Can you work these out from the drawing? Everything is in mm from the part's minimum corner. Round coordinates to 2 decimals unless told otherwise and drop trailing zeros. Loops run counter-clockwise (first coordinate to the right, second up) from the corner with the lowest first, then second, coordinate; pieces in that order, holes last. Notation, with made-up numbers: (82.5, 39) -> (134.5, 39) arc R34 cw to (134.5, 72) -> close; hole circle Ø10 at (40, -33.75). An arc over 180 degrees is marked (long way). One line per item, written item: value.
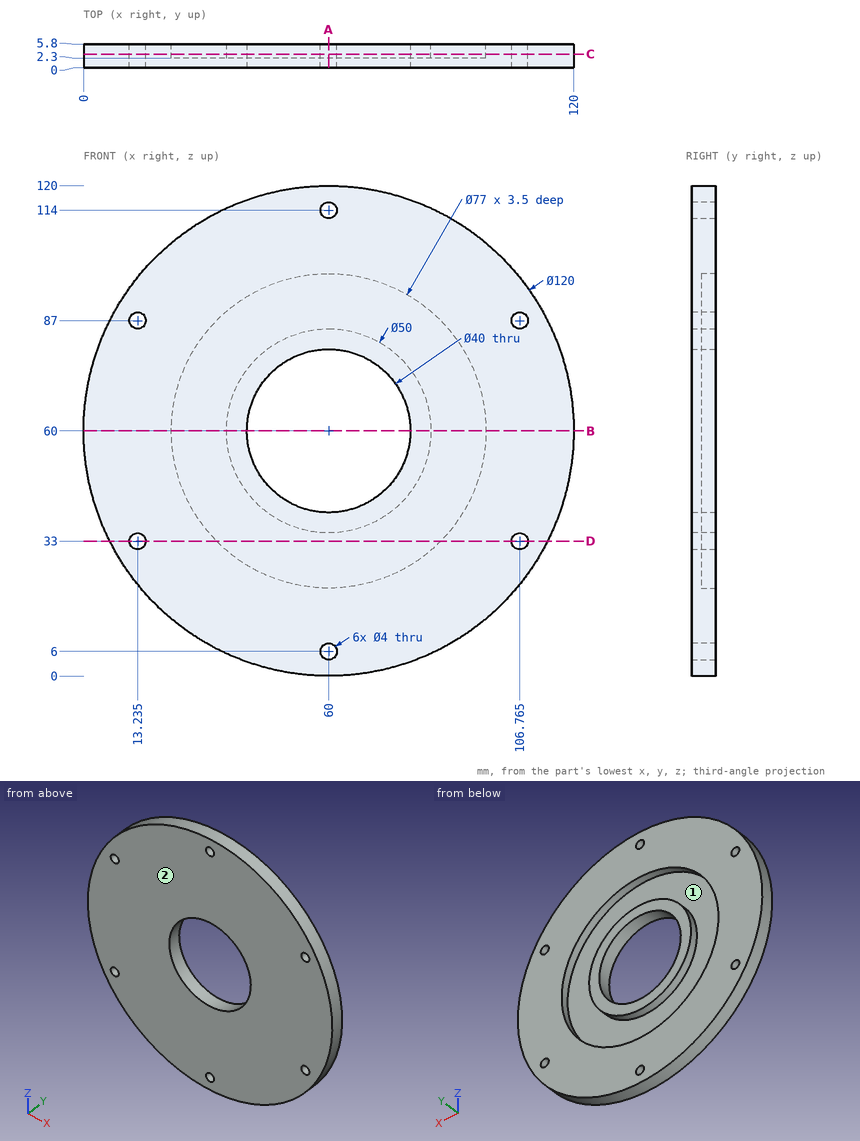
(1) Thinking about a two-plate mould opening in X: for the marked faces 1 and 2, which applies, released by +X, released by -X, zero draft, split by the parting line, or undercut?
Recorded:
face 1: undercut
face 2: zero draft
(2) If I drill on L1, parallel to X at y = 3.55, z = 60.5 (1 decimal); L2, parallel to X at y = 3.8, z = 37 (1 decimal); L3, parallel to X at y = 3.2, z = 87 (1 decimal), over which ranges is the centre line in solid material (lowest first)?
Recorded:
L1: 0 to 21.5, 35 to 40, 80 to 85, 98.5 to 120
L2: 4.6 to 29.1, 50.2 to 69.8, 90.9 to 115.4
L3: 6.4 to 11.2, 15.2 to 32.6, 87.4 to 104.8, 108.8 to 113.6
(3) If we section it at A-A, the plane x = 60: Please give me the cut outline in (y, z), then the cut area to 3 significant figures.
Recorded:
outline: (0, 0) -> (5.8, 0) -> (5.8, 4) -> (0, 4) -> close; (0, 8) -> (5.8, 8) -> (5.8, 21.5) -> (2.3, 21.5) -> (2.3, 35) -> (5.8, 35) -> (5.8, 40) -> (0, 40) -> close; (0, 80) -> (5.8, 80) -> (5.8, 85) -> (2.3, 85) -> (2.3, 98.5) -> (5.8, 98.5) -> (5.8, 112) -> (0, 112) -> close; (0, 116) -> (5.8, 116) -> (5.8, 120) -> (0, 120) -> close
area: 323 mm²
(4) If we section it at D-D, the plane z = 33: Please give me the cut outline in (x, y) (1 decimal), then the cut area to 3 significant figures.
Recorded:
outline: (6.4, 0) -> (11.2, 0) -> (11.2, 5.8) -> (6.4, 5.8) -> close; (15.2, 0) -> (104.8, 0) -> (104.8, 5.8) -> (87.4, 5.8) -> (87.4, 2.3) -> (32.6, 2.3) -> (32.6, 5.8) -> (15.2, 5.8) -> close; (108.8, 0) -> (113.6, 0) -> (113.6, 5.8) -> (108.8, 5.8) -> close
area: 383 mm²
(5) If we section it at B-B, the plane z = 60: Please give me the cut outline in (x, y).
Recorded:
outline: (0, 0) -> (40, 0) -> (40, 5.8) -> (35, 5.8) -> (35, 2.3) -> (21.5, 2.3) -> (21.5, 5.8) -> (0, 5.8) -> close; (80, 0) -> (120, 0) -> (120, 5.8) -> (98.5, 5.8) -> (98.5, 2.3) -> (85, 2.3) -> (85, 5.8) -> (80, 5.8) -> close
(6) If we section it at C-C, the plane y = 3.35: Give the number of separate pieces and of enclosed holes in the cut face.
Recorded:
separate pieces: 2
enclosed holes: 8
(7) I'm going to push flat-ended pins straight in: pin 1 Ø2 at (x, y) = (72, 1.5) entering from -Z; pin 2 Ø3 at (x, z) = (13.23, 87) entering from +Y; pin 3 Ø1 at (x, y) = (20.5, 1) entering from +Z (1 decimal); pin 4 Ø3 at (y, z) = (4, 27) entering from +X. Where does each tip first touch, or does it pass through?
Recorded:
pin 1: z = 1.02
pin 2: through
pin 3: z = 105.6
pin 4: x = 111.07
